Input: part model. Units: mm. Frame: model coordinates. A direction names the side the tool comes from. Give positions to 0.01 mm unless a question says otherwise; leave off trailing zeros. Write each loop counter-clockwise with the first axis right and the second up, starting at its lowest first coordinate (ties: lowest second). Pieces come first, ordered by that corner, then holes. Notation, with made-up numbers: (84.5, 71) -> (105.5, 71) arc R32 ccw to (105.5, 106) -> close; hole circle Ø4 at (-23, -27.5). An arc over 180 degrees is marked (long way). Return JSON: item names as keys, results as strings. Group by question number.
Item 1: Mould query, pull axis X, two halves, no side actions, for faces 4 (the face through (39.003, 9.382, 0.986)), 5 (the face through (-1, 0, 0)), 6 (the face through (20.74, 21.9, 21.8)). Classes: released by +X, released by -X, zero draft, split by the parting line, or undercut.
Item 2: Pin query (flat end, axial travel): P1, Ø1.5, axis at y = 9, z = 25, coming from the +X side; P2, Ø12, axis at x = 16, y = 17.5, coming from the +Z side; P3, Ø15, axis at x = 56.5, y = 1.5, coming from the +Z side; P4, Ø12, axis at y = -0.5, z = 17, coming from the -X side. Return the tip coordinate at first contact, or that it passes through.
Item 3: Line query: line 1 (Y direction, x = 66, z = 1.45); line 2 (X direction, y = -9, z = 1); line 3 (Z direction, x = -46, y = 11). Output: solid intervals per line, ascending. Write a range as [from, to].
Item 4: Section A-A, the plane x = 42. Return loops of the section in (y, z).
Item 5: Set-up query: faces 1 (the face through (19.765, -0.328, 5.451)), 2 (the face through (-39.3, 15, 1.8)), 3 (the face through (25, -5, 20)). Return all of +Z, -Z, +X, -X, +Y, -Y with unobstructed straight access to the full face (end or side cutting, diameter ignored); none if empty.
Item 6: Section B-B, the plane y = 9.25. Count the separate pieces of the cut face and the enclosed holes in it, then the cut area to 3 significant figures.
from build123d import *

# Parameters (mm, degrees)
F0_R         = 3
F1_DEPTH     = 2
F3_DEPTH     = 21
F4_R         = 2
F5_DEPTH     = 3
F6_DEPTH     = 44.001
F7_SIZE      = 7
F8_DEPTH     = 13
F9_SIZE      = 26
F10_T1_DEPTH = 54.8534078581
F10_T3_DEPTH = 54.8534078581
F11_SIZE     = 8
F12_SIZE     = 1
F13_SIZE     = 1
F14_R        = 1.2
F15_DEPTH    = 2


# Not quite as in the source:
# - a fillet or chamfer that OpenCascade refuses, or shapes differently, is made with other operations: its cross-section is extruded or revolved along the edge and cut away or added


with BuildPart() as f1:
    # F0 (on Top) → F1 (new body)
    with BuildSketch(Plane.XY):
        Polygon((-71, -15), (71, -15), (71, 15), (26.313708499, 15), (15, 29), (-15, 29), (-26.313708499, 15), (-71, 15), align=None)
        with Locations((-66, -9.25)):
            Circle(F0_R, mode=Mode.SUBTRACT)
        with Locations((-42, -9.25)):
            Circle(F0_R, mode=Mode.SUBTRACT)
        with Locations((42, -9.25)):
            Circle(F0_R, mode=Mode.SUBTRACT)
        with Locations((66, -9.25)):
            Circle(F0_R, mode=Mode.SUBTRACT)
        with Locations((-66, 9.25)):
            Circle(F0_R, mode=Mode.SUBTRACT)
        with Locations((-42, 9.25)):
            Circle(F0_R, mode=Mode.SUBTRACT)
        with Locations((42, 9.25)):
            Circle(F0_R, mode=Mode.SUBTRACT)
        with Locations((66, 9.25)):
            Circle(F0_R, mode=Mode.SUBTRACT)
    extrude(amount=F1_DEPTH)

    # F2 (on face) → F3 (join)
    with BuildSketch(Plane.XY.offset(2)):
        Polygon((-15, 29), (-26.313708499, 15), (-26.313708499, -15), (-23.313708499, -15), (-23.313708499, 13.9393398282), (-13.5672232498, 26), (13.5672232498, 26), (23.313708499, 13.9393398282), (23.313708499, -15), (26.313708499, -15), (26.313708499, 15), (15, 29), align=None)
    extrude(amount=F3_DEPTH)

    # F4 (on face) → F5 (join)
    with BuildSketch(Plane(origin=(0, 29, 0), x_dir=(-1, 0, 0), z_dir=(0, 1, 0))):
        with BuildLine():
            ThreePointArc((-4.75, 23), (0, 27.75), (4.75, 23))
            Line((4.75, 23), (15, 23))
            Line((15, 23), (15, 36))
            Line((15, 36), (0, 36))
            Line((0, 36), (-15, 36))
            Line((-15, 36), (-15, 23))
            Line((-15, 23), (-4.75, 23))
        make_face()
        with Locations((-8.2078662679, 27.7834016482)):
            Circle(F4_R, mode=Mode.SUBTRACT)
        with Locations((8.2464804778, 27.7165198748)):
            Circle(F4_R, mode=Mode.SUBTRACT)
    extrude(amount=-F5_DEPTH)

    # F4 (on face) → F6 (cut, through all)
    with BuildSketch(Plane(origin=(0, 29, 0), x_dir=(-1, 0, 0), z_dir=(0, 1, 0))):
        with Locations((-8.2078662679, 27.7834016482)):
            Circle(F4_R)
        with BuildLine():
            ThreePointArc((-4.75, 23), (0, 18.25), (4.75, 23))
            Line((4.75, 23), (-4.75, 23))
        make_face()
        with Locations((-0.0386142099, 13.500078477)):
            Circle(F4_R)
    extrude(amount=-F6_DEPTH, mode=Mode.SUBTRACT)

    # F7
    f7_edges = [f1.edges().sort_by_distance(p)[0] for p in [
        (-26.313708, 0, 2),
        (23.313708, -0.53033, 2),
        (18.440466, 19.96967, 2),
        (-18.440466, 19.96967, 2),
        (-23.313708, -0.53033, 2),
        (26.313708, 0, 2),
        (0, 26, 2),
        (0, 29, 0),
    ]]
    chamfer(f7_edges, length=F7_SIZE)

    # F8 (add): faces of the model
    f8_faces = [f1.faces().sort_by_distance(p)[0] for p in [
        (-15.4580909174, 27.5, 23),
        (25.8556175816, 0, 23),
    ]]
    extrude(f8_faces, amount=F8_DEPTH)

    # F9
    f9_edges = [f1.edges().sort_by_distance(p)[0] for p in [
        (-24.813708, -15, 36),
        (24.813708, -15, 36),
    ]]
    chamfer(f9_edges, length=F9_SIZE)

    # F10: chamfer of 10 on 2 edges, made by hand

    # F10_s2 → F10_t1 (cut)
    with BuildSketch(Plane.YZ.offset(-52.2404124281)):
        Polygon((3.9289321881, 28.9289321881), (21, 36), (11, 36), align=None)
    extrude(amount=F10_T1_DEPTH, mode=Mode.SUBTRACT)

    # F10_s4 → F10_t3 (cut)
    with BuildSketch(Plane.YZ.offset(-2.6129954301)):
        Polygon((3.9289321881, 28.9289321881), (21, 36), (11, 36), align=None)
    extrude(amount=F10_T3_DEPTH, mode=Mode.SUBTRACT)

    # F11
    f11_edges = [f1.edges().sort_by_distance(p)[0] for p in [
        (23.485281, 18.5, 0),
        (-23.485281, 18.5, 0),
    ]]
    chamfer(f11_edges, length=F11_SIZE)

    # F12
    f12_edges = [f1.edges().sort_by_distance(p)[0] for p in [
        (2.038614, 29, 13.500078),
        (10.207866, 29, 27.783402),
        (-6.24648, 29, 27.71652),
    ]]
    chamfer(f12_edges, length=F12_SIZE)

    # F13
    f13_edges = [f1.edges().sort_by_distance(p)[0] for p in [
        (-4.75, 26, 23),
        (-4.75, 29, 23),
    ]]
    chamfer(f13_edges, length=F13_SIZE)

    # F14 (on face) → F15 (cut, through all)
    with BuildSketch(Plane(origin=(0, 0, 0), x_dir=(1, 0, 0), z_dir=(0, 0, -1))):
        with Locations((-4.75, -17)):
            Circle(F14_R)
        with BuildLine():
            ThreePointArc((5.95, -17), (4.75, -15.8), (3.55, -17))
            ThreePointArc((3.55, -17), (4.75, -18.2), (5.95, -17))
        make_face()
    extrude(amount=-F15_DEPTH, mode=Mode.SUBTRACT)


solid = f1.part
Answer below:
{
 "1": {"face 4": "undercut", "face 5": "zero draft", "face 6": "released by +X"},
 "2": {"P1": "stops at x = 26.31", "P2": "stops at z = 36", "P3": "stops at z = 2", "P4": "stops at x = -26.31"},
 "3": {"line 1": "y = [-15, -12.25], [-6.25, 6.25], [12.25, 15]", "line 2": "x = [-71, -68.99], [-63.01, -44.99], [-39.01, 39.01], [44.99, 63.01], [68.99, 71]", "line 3": "z = [0, 2]"},
 "4": {"outline": "(-15, 0) -> (-12.25, 0) -> (-12.25, 2) -> (-15, 2) -> close; (-6.25, 0) -> (6.25, 0) -> (6.25, 2) -> (-6.25, 2) -> close; (12.25, 0) -> (15, 0) -> (15, 2) -> (12.25, 2) -> close"},
 "5": {"face 1": "+Z, -Y", "face 2": "-Z, -X, +Y", "face 3": "+Z, +X, -X, -Y"},
 "6": {"separate pieces": "5", "enclosed holes": "0", "area": "509 mm2"}
}
